from build123d import *

# Parameters (mm, degrees)
F0_W     = 50
F0_H     = 30
F1_DEPTH = 6
F3_D     = 6.6
F3_DEPTH = 15
F3_TIP   = 1.9828400428
F4_SIZE  = 1


with BuildPart() as f1:
    # F0 (on Front) → F1 (new body, symmetric)
    with BuildSketch(Plane.XZ):
        Rectangle(F0_W, F0_H)
    extrude(amount=F1_DEPTH, both=True)

    # F3
    with Locations(Plane(origin=(0, 0, -15), x_dir=(1, 0, 0), z_dir=(0, 0, -1))):
        with Locations((-15, 0), (15, 0)):
            Hole(F3_D / 2, depth=F3_DEPTH)
            with Locations((0, 0, -(F3_DEPTH + F3_TIP / 2))):  # 118° drill point
                Cone(0, F3_D / 2, F3_TIP, mode=Mode.SUBTRACT)

    # F4
    f4_edges = [f1.edges().sort_by_distance(p)[0] for p in [
        (0, -6, -15),
        (25, -6, 0),
        (0, -6, 15),
        (-25, -6, 0),
        (25, 0, 15),
        (0, 6, 15),
        (-25, 0, 15),
        (25, 0, -15),
        (25, 6, 0),
        (0, 6, -15),
        (-25, 6, 0),
        (-25, 0, -15),
        (-18.3, 0, -15),
        (11.7, 0, -15),
    ]]
    chamfer(f4_edges, length=F4_SIZE)


solid = f1.part
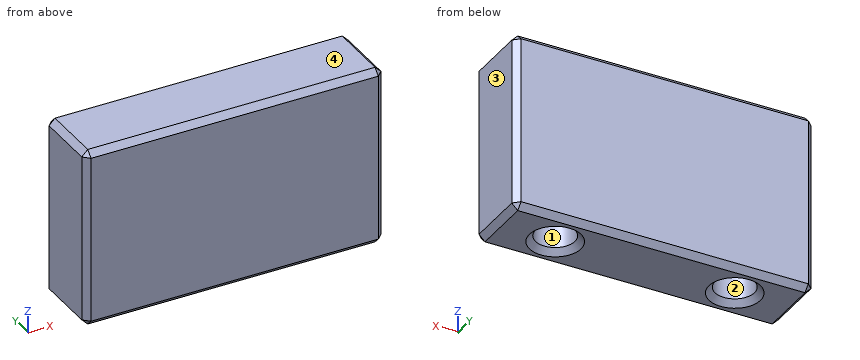
Could you check a few things on this model? Use its own coordinates, in mm. Face numbers are marked on the shaded views. Coordinates: 2 decimals unless noted, no trailing zeros. Loops run counter-clockwise (first coordinate to the right, second up) from the corner with the lowest first, then second, coordinate; pieces in that order, holes last. Notation, with made-up numbers: (79, 5.25) -> (129, 5.25) arc R20 ccw to (129, 22.25) -> close; hole circle Ø7 at (17.25, 35.5). An arc over 180 degrees is marked (long way). Answer in a Markdown table with one row per item.
(1) Imagine slicing it at A-A (z = -2.25). List the corners of the cut face in (x, y) for me, plus the area to 3 significant figures.
Results found:
| item | result |
|---|---|
| outline | (-25, -5) -> (-24, -6) -> (24, -6) -> (25, -5) -> (25, 5) -> (24, 6) -> (-24, 6) -> (-25, 5) -> close; hole circle Ø6.6 at (-15, 0); hole circle Ø6.6 at (15, 0) |
| area | 530 mm^2 |
(2) Thinking about a two-plate mould opening in X: for the marked faces 1, 2, 3 and 4, which applies, released by +X, released by -X, zero draft, split by the parting line, or undercut?
Results found:
| item | result |
|---|---|
| face 1 | undercut |
| face 2 | undercut |
| face 3 | released by +X |
| face 4 | zero draft |
(3) Will this pin go through, and if not, where does the flat tip stop? pin 1 Ø6 at (x, y) = (-15, 0) entering from -Z.
Results found:
| item | result |
|---|---|
| pin 1 | stops at z = 0.18 |
(4) If I drill on probe 1 along X at (y, z) = (0, -3.5); probe 2 along Y at (x, z) = (15, -4); probe 3 along X at (y, z) = (2.25, -6), over which ranges is the centre line in solid material (lowest first)?
Results found:
| item | result |
|---|---|
| probe 1 | x = -25 to -18.3, -11.7 to 11.7, 18.3 to 25 |
| probe 2 | y = -6 to -3.3, 3.3 to 6 |
| probe 3 | x = -25 to -17.41, -12.59 to 12.59, 17.41 to 25 |
